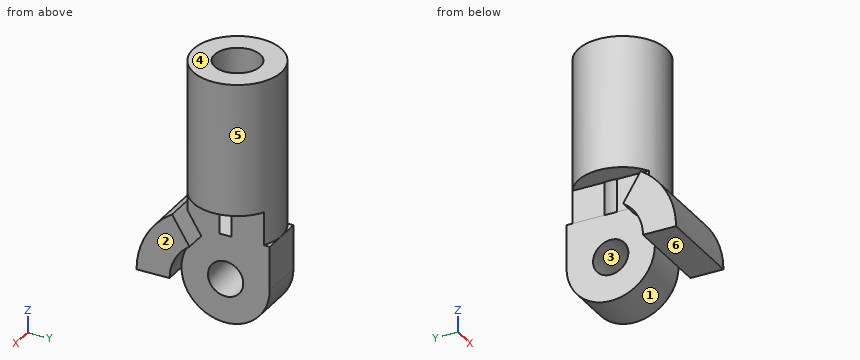
Autodesk Inventor part; units mm, degrees
ref_plane "YZ Plane" through (0, 0, 0) normal (1, 0, 0) x (0, 1, 0)
ref_plane "XZ Plane" through (0, 0, 0) normal (0, 1, 0) x (-1, 0, 0)
ref_plane "XY Plane" through (0, 0, 0) normal (0, 0, 1) x (1, 0, 0)
sketch "Sketch1" plane through (0, 0, 0) normal (0, 0, 1) x (1, 0, 0)
  circle A0 centre (0, 0) radius 2
  circle A1 centre (0, 0) radius 4
  dimension "d0" = 4
  dimension "d1" = 8
extrude "Extrusion1" add sketch "Sketch1" along normal blind 15
sketch "Sketch2" plane through (0, 0, 0) normal (0, 0, -1) x (-1, 0, 0)
  circle A0 centre (0, 0) radius 4
  line L0 (0, 4) -> (4, 4)
  line L1 (4, 4) -> (4, -4)
  line L2 (4, -4) -> (0, -4)
  line L3 (0, -4) -> (0, 4)
  line L4 (4, -4) -> (-4, -4)
  line L5 (-4, -4) -> (-4, 4)
  line L6 (-4, 4) -> (4, 4)
  line L7 (4, 4) -> (4, -4)
extrude "Extrusion2" add sketch "Sketch2" along normal blind 8
sketch "Sketch3" plane through (4, 0, 0) normal (1, 0, 0) x (0, 0, -1)
  circle A0 centre (4, 0) radius 4
  line L0 (0, 4) -> (0, 0)
  line L1 (8, 4) -> (8, -4)
  line L2 (0, 4) -> (8, 4)
  line L3 (8, 4) -> (8, -4)
  line L4 (8, -4) -> (0, -4)
  line L5 (0, -4) -> (0, 4)
  point P0 (4, -4)
  point P1 (8, 0)
  point P2 (4, 4)
extrude "Extrusion3" cut sketch "Sketch3" against normal blind 8 contours L1 L4 A0 | A0 L2 L1
sketch "Sketch4" plane through (4, 0, 0) normal (1, 0, 0) x (0, 0, -1)
  circle A0 centre (4.0004, 0) radius 1.6
  point P0 (0, 0)
  dimension "d8" = 3.2
extrude "Extrusion4" cut sketch "Sketch4" against normal blind 8
sketch "Sketch5" plane through (0, 0, 0) normal (0, 0, 1) x (1, 0, 0)
  line L0 (0, 4) -> (4, 4)
  line L1 (0, -4) -> (-4, -4)
  line L2 (2, 4) -> (-2, 4)
  line L3 (-2, 4) -> (-2, -4)
  line L4 (-2, -4) -> (2, -4)
  line L5 (2, -4) -> (2, 4)
  line L6 (4, -4) -> (0, -4)
  line L7 (4, -4) -> (-4, -4)
  line L8 (-4, -4) -> (-4, 4)
  line L9 (-4, 4) -> (4, 4)
  line L10 (4, 4) -> (4, -4)
  point P0 (0, 0)
extrude "Extrusion5" cut sketch "Sketch5" against normal blind 8 contours L0 L10 L6 L5 | L3 L1 L8 L9
sketch "Sketch6" plane through (0, -4, 0) normal (0, -1, 0) x (1, 0, 0)
  line L0 (-2, -4) -> (2, -4)
  line L1 (-2, 0) -> (-4, 0)
  line L2 (0, -4) -> (-4, -4)
  line L3 (-4, -4) -> (-4, 0)
  line L4 (-4, 0) -> (0, 0)
  line L5 (0, 0) -> (0, -4)
  line L6 (0, -4) -> (3.9704, -4)
  line L7 (3.9704, -4) -> (3.9704, 0)
  line L8 (3.9704, 0) -> (0, 0)
  line L9 (0, 0) -> (0, -4)
extrude "Extrusion6" add sketch "Sketch6" along normal blind 3
sketch "Sketch7" plane through (0, 0, 0) normal (0, 0, -1) x (-1, 0, 0)
  line L0 (2, 4) -> (-2, 4)
  line L1 (-2, -4) -> (-2, 4)
  line L2 (2, 4) -> (-2, 4)
  line L3 (-2, 4) -> (-2, -4)
  line L4 (-2, -4) -> (2, -4)
  line L5 (2, -4) -> (2, 4)
  line L6 (5.0463, 4) -> (-4.8372, 4)
  line L7 (-4.8372, 4) -> (-4.8372, -4)
  line L8 (-4.8372, -4) -> (5.0463, -4)
  line L9 (5.0463, -4) -> (5.0463, 4)
  point P0 (0, 0)
extrude "Extrusion7" cut sketch "Sketch7" against normal blind 3 contours L6 L9 L8 L5 | L1 L8 L7 L6
sketch "Sketch8" plane through (-2, 3.4641, 0) normal (-1, 0, 0) x (0, 0, 1)
  circle A0 centre (-3.9998, -3.4641) radius 4
  circle A1 centre (-3.9998, -3.4641) radius 6.9959
  line L0 (-0.6612, -5.6672) -> (1.8871, -7.244)
  line L1 (-3.9998, -7.4641) -> (-3.9998, -10.46)
  circle A2 centre (-3.9998, -3.4641) radius 8.7454
  line L2 (0.613, -8.7238) -> (1.7591, -10.0457)
  line L3 (-5.354, -10.3276) -> (-5.7862, -12.0251)
  point P0 (0, -3.4641)
extrude "Extrusion8" cut sketch "Sketch8" along normal mid plane 20 contours A1 L2 A2 L3 picked at (0.8234, -9.9865)
extrude "Extrusion9" add sketch "Sketch8" along normal blind 2 and the other way blind 6 contours A0 L0 A1 L1 picked at (-3.4455, -9.3945)
sketch "Sketch9" plane through (0, 0, 15) normal (0, 0, 1) x (1, 0, 0)
  arc A0 (2, 0) -> (-2, 0) centre (0, 0) ccw
  circle A1 centre (0, 0) radius 2.075
  dimension "d23" = 4.15
extrude "Extrusion10" cut sketch "Sketch9" against normal blind 15
properties part number "hingejoint1"
The model under review builds one solid part; all positions refer to its coordinate system, in mm. Face numbers are marked on the shaded views. A direction names the side the tool comes from. Round coordinates to 2 decimals unless told otherwise and drop trailing zeros. Loops run counter-clockwise (first coordinate to the right, second up) from the corner with the lowest first, then second, coordinate; pieces in that order, holes last. Notation, with made-up numbers: (40.5, 26) -> (64.5, 26) arc R34 ccw to (64.5, 59) -> close; hole circle Ø11 at (41.5, 52). An arc over 180 degrees is marked (long way). Answer as CSV lines item,"result".
1) To check wall thickness, follow line 1 along Y through (x, z) = (0, 8.5) (3 decimals); line 2 along X through (y, z) = (2.25, -0.75); line 3 along X through (y, z) = (1.75, 5). State the ranges of each line that lie inside material, in increasing order. Write a range as from..to.
Geometry results:
line 1,"y = -4..-2.075, 2.075..4"
line 2,"x = -2..2"
line 3,"x = -3.6..-1.11, 1.11..3.6"
2) For P1, Ø4, axis at y = -4, z = 10.5, coming from the +X side; P2, Ø1.5, axis at x = -3, z = -0.5, coming from the -Y side; P3, Ø1.6, axis at x = 2.5, y = 1.5, coming from the -Z side; P4, Ø2.5, axis at y = 0, z = -4, coming from the -X side, all flat-tipped, find the tip position at first contact; note any pin that passes through.
Geometry results:
P1,"stops at x = 3.46"
P2,"stops at y = -6.43"
P3,"stops at z = -7.9"
P4,"passes through"
3) Add section B-B on y = 0. Write out the cut boundary in (x, z) (3 decimals), plus the area to 3 significant figures.
Geometry results:
outline,"(-4, 3) -> (-2.075, 3) -> (-2.075, 15) -> (-4, 15) -> close; (-2, -8) -> (2, -8) -> (2, -5.6) -> (-2, -5.6) -> close; (-2, -2.4) -> (2, -2.4) -> (2, 0) -> (-2, 0) -> close; (2.075, 3) -> (4, 3) -> (4, 15) -> (2.075, 15) -> close"
area,"65.4 mm²"
4) Add section C-C on y = 1.25. Write out the cut boundary in (x, z), plus the area to 3 significant figures.
Geometry results:
outline,"(-3.8, 3) -> (-2, 3) -> (-2, -3) -> (2, -3) -> (2, 3) -> (3.8, 3) -> (3.8, 15) -> (1.66, 15) -> (1.66, 0) -> (-1.66, 0) -> (-1.66, 15) -> (-3.8, 15) -> close; (-2, -7.8) -> (2, -7.8) -> (2, -5) -> (-2, -5) -> close"
area,"76.7 mm²"
5) Add section D-D on x = -1.75. Write out the cut boundary in (y, z), plus the area to 3 significant figures.
Geometry results:
outline,"(-7, -4) -> (-4, -4) arc R4 ccw to (4, -4) -> (4, 0) -> (3.6, 0) -> (3.6, 15) -> (1.11, 15) -> (1.11, 0) -> (-1.11, 0) -> (-1.11, 15) -> (-3.6, 15) -> (-3.6, 1.59) -> (-3.78, 1.89) arc R7 ccw to start; hole circle Ø3.2 at (0, -4)"
area,"136 mm²"
6) Add section A-A on z = 2.5. Write out the cut boundary in (x, y) (3 decimals), plus the area to 3 significant figures.
Geometry results:
outline,"(-2, -3.464) arc R4 ccw to (2, -3.464) -> (2, -0.553) arc R2.075 cw to (-2, -0.553) -> close; (-2, 0.553) arc R2.075 cw to (2, 0.553) -> (2, 3.464) arc R4 ccw to (-2, 3.464) -> close"
area,"17.2 mm²"
7) Tool access review of the marked faces 4, 5 and 6: name each direction out of +Z, -Z, +X, -X, +Y, -Y from which nothing blocks a thin tool from reaching the whole face with its end or side.
Geometry results:
face 4,"+Z, +X, -X, +Y, -Y"
face 5,"+Z"
face 6,"-Z, +X, -X, -Y"
8) Draft analysis for pull direction Y (two halves, no side actions). For the marked faces 1, 2 and 3, state which applies: pulls with the +Y half, pulls with the -Y half, needs draft (parallel to the pull), parting line crosses it, or undercut.
Geometry results:
face 1,"parting line crosses it"
face 2,"needs draft"
face 3,"undercut"
